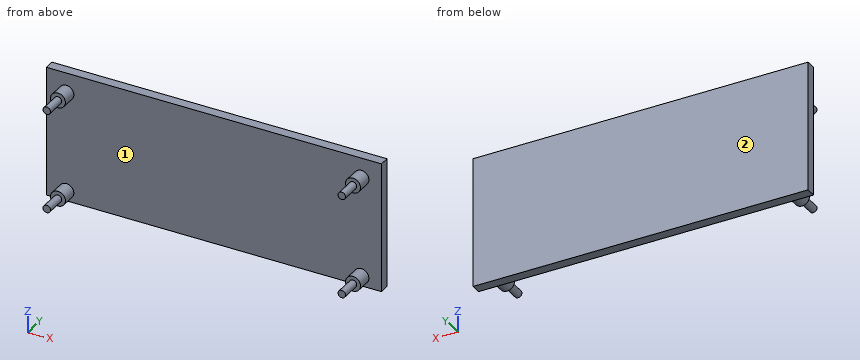
Autodesk Fusion 360 part; units mm, degrees
sketch "Sketch1" plane through (0, 0, 0) normal (0, 1, 0) x (1, 0, 0)
  line L0 (0, 0) -> (67, 0)
  line L1 (67, 0) -> (67, -26)
  line L2 (67, -26) -> (0, -26)
  line L3 (0, -26) -> (0, 0)
  dimension "d1" = 67
  dimension "d2" = 26
extrude "Extrude1" add sketch "Sketch1" along normal blind 2
sketch "Sketch2" plane through (0, 0, 0) normal (0, 1, 0) x (1, 0, 0)
  circle A0 centre (4, -2) radius 1.5
  circle A1 centre (63, -2) radius 1.5
  circle A2 centre (4, -22) radius 1.5
  circle A3 centre (63, -22) radius 1.5
  dimension "d5" = 3
  dimension "d6" = 3
  dimension "d7" = 3
  dimension "d8" = 3
extrude "Extrude2" add sketch "Sketch2" against normal blind 3
sketch "Sketch3" plane through (0, 0, 0) normal (0, 1, 0) x (1, 0, 0)
  circle A0 centre (4, -22) radius 0.75
  circle A1 centre (4, -2) radius 0.75
  circle A2 centre (63, -22) radius 0.75
  circle A3 centre (63, -2) radius 0.75
  dimension "d11" = 1.5
  dimension "d12" = 1.5
  dimension "d13" = 1.5
  dimension "d14" = 1.5
extrude "Extrude3" add sketch "Sketch3" against normal blind 7 contours A0
sketch "Sketch4" plane through (0, 0, 0) normal (0, 1, 0) x (1, 0, 0)
  circle A0 centre (4, -2) radius 0.75
  dimension "d17" = 1.5
extrude "Extrude4" add sketch "Sketch4" against normal blind 7
sketch "Sketch5" plane through (0, 0, 0) normal (0, 1, 0) x (1, 0, 0)
  circle A0 centre (63, -22) radius 0.75
  dimension "d20" = 1.5
extrude "Extrude5" add sketch "Sketch5" against normal blind 7
sketch "Sketch6" plane through (0, 0, 0) normal (0, 1, 0) x (1, 0, 0)
  circle A0 centre (63, -2) radius 0.75
  dimension "d23" = 1.5
extrude "Extrude6" add sketch "Sketch6" against normal blind 7
Can you work these out from the model? Positions are in its coordinate system, mm. Face numbers are marked on the shaded views. Coordinates: 2 decimals unless noted, no trailing zeros. Write each loop counter-clockwise with the first axis right and the second up, starting at its lowest first coordinate (ties: lowest second). Pieces come first, ordered by that corner, then holes. Notation, with made-up numbers: M -6,66 L 4,66 A27 ccw 4,99 Z; hole C -37,-30 d7. An arc over 180 degrees is marked long. Answer as CSV lines item,"result".
Item 1: Please list where these lines run through material, in increasing order: line 1 along X through (y, z) = (-1.75, 22); line 2 along Y through (x, z) = (28, 7.25); line 3 along Z through (x, y) = (62, -2.25).
Geometry results:
line 1,"x = 2.5 to 5.5, 61.5 to 64.5"
line 2,"y = 0 to 2"
line 3,"z = 0.88 to 3.12, 20.88 to 23.12"
Item 2: Imagine slicing it at B-B on x = 4. List the corners of the cut face in (y, z) for me, plus the area to 3 significant figures.
Geometry results:
outline,"M -7,1.25 L -3,1.25 L -3,0.5 L 0,0.5 L 0,0 L 2,0 L 2,26 L 0,26 L 0,23.5 L -3,23.5 L -3,22.75 L -7,22.75 L -7,21.25 L -3,21.25 L -3,20.5 L 0,20.5 L 0,3.5 L -3,3.5 L -3,2.75 L -7,2.75 Z"
area,"82.0 mm2"
Item 3: Imagine slicing it at C-C on x = 30. List the corners of the cut face in (y, z) for me, plus the area to 3 significant figures.
Geometry results:
outline,"M 0,0 L 2,0 L 2,26 L 0,26 Z"
area,"52.0 mm2"
Item 4: I'm going to push a flat-ended pin straight in: P1, Ø8, axis at x = 38, z = 17, coming from the -Y side. Where does the tip first touch, or does it pass through?
Geometry results:
P1,"stops at y = 0"
Item 5: Imagine slicing it at A-A on z = 2. List the corners of the cut face in (x, y) for me.
Geometry results:
outline,"M 0,0 L 2.5,0 L 2.5,-3 L 3.25,-3 L 3.25,-7 L 4.75,-7 L 4.75,-3 L 5.5,-3 L 5.5,0 L 61.5,0 L 61.5,-3 L 62.25,-3 L 62.25,-7 L 63.75,-7 L 63.75,-3 L 64.5,-3 L 64.5,0 L 67,0 L 67,2 L 0,2 Z"
Item 6: We'd pull the mould along X, two halves only. Please class the marked faces 1 and 2: +X half, -X half, draft (parallel to the pull), parting line (faces both ways), or undercut.
Geometry results:
face 1,"undercut"
face 2,"draft"
